```python
from build123d import *

# Parameters (mm, degrees)
SKETCH1_W           = 13
SKETCH1_H           = 8.9
BOSS_EXTRUDE1_DEPTH = 2
SKETCH2_R           = 1.75
CUT_EXTRUDE4_DEPTH  = 9.127268914
SKETCH3_R           = 2.95
CUT_EXTRUDE9_DEPTH  = 0.5
CHAMFER1_SIZE       = 0.5
FILLET2_R           = 2


with BuildPart() as part:
    # Sketch1 → Boss-Extrude1 (new body)
    with BuildSketch(Plane.XY):
        Rectangle(SKETCH1_W, SKETCH1_H)
    extrude(amount=BOSS_EXTRUDE1_DEPTH)

    # Sketch2 → Cut-Extrude4 (cut, through all)
    with BuildSketch(Plane.XY.offset(2)):
        with Locations((-0.4, 1.45)):
            Circle(SKETCH2_R)
    extrude(amount=-CUT_EXTRUDE4_DEPTH, mode=Mode.SUBTRACT)

    # Sketch3 → Cut-Extrude9 (cut)
    with BuildSketch(Plane.XY.offset(2)):
        with Locations((-0.4, 1.45)):
            Circle(SKETCH3_R)
    extrude(amount=-CUT_EXTRUDE9_DEPTH, mode=Mode.SUBTRACT)

    # Chamfer1
    chamfer1_edges = [part.edges().sort_by_distance(p)[0] for p in [
        (-2.15, 1.45, 0),
        (0, -4.45, 0),
        (-6.5, 0, 0),
        (0, 4.45, 0),
        (6.5, 0, 0),
    ]]
    chamfer(chamfer1_edges, length=CHAMFER1_SIZE)

    # Fillet2
    # the kernel refuses this fillet: 2 mm, written as the material it takes off along each edge
    with BuildSketch(Plane(origin=(-6.5, 4.45, -4.5), x_dir=(0, -1, 0), z_dir=(0, 0, 1)), Plane(origin=(-6.5, -4.45, -4.5), x_dir=(1, 0, 0), z_dir=(0, 0, 1))) as fillet2_piece_1:
        with BuildLine():
            CenterArc((FILLET2_R, FILLET2_R), FILLET2_R, 180, 90)
            Line((0, FILLET2_R), (0, 0))
            Line((0, 0), (FILLET2_R, 0))
        make_face()
    extrude(amount=11.5, mode=Mode.SUBTRACT)
    with BuildSketch(Plane(origin=(6.5, 4.45, -4.5), x_dir=(0, -1, 0), z_dir=(0, 0, 1)), Plane(origin=(6.5, -4.45, -4.5), x_dir=(-1, 0, 0), z_dir=(0, 0, 1))) as fillet2_piece_2:
        with BuildLine():
            CenterArc((FILLET2_R, -FILLET2_R), FILLET2_R, 90, 90)
            Line((0, -FILLET2_R), (0, 0))
            Line((0, 0), (FILLET2_R, 0))
        make_face()
    extrude(amount=11.5, mode=Mode.SUBTRACT)


solid = part.part
```
Design review of the part built by this model. Coordinates are the model's own, in mm. Give positions to 0.01 mm unless a question says otherwise; leave off trailing zeros. Loops run counter-clockwise (first coordinate to the right, second up) from the corner with the lowest first, then second, coordinate; pieces in that order, holes last. Notation, with made-up numbers: M 34,77.5 L 92,77.5 A14 ccw 92,85.5 Z; hole C 89.5,-13 d7. An arc over 180 degrees is marked long. Return JSON: item names as keys, results as strings. Group by question number.
Item 1: We need section C-C (x = -0.4). Give the boundary of the cut face in (y, z).
Item 2: We need section A-A (y = 1.45). Give the boundary of the cut face in (x, z).
Item 3: Mouldability with a two-part tool opening along X and no side actions: class faces 1 (the cylindrical face through (5.93, 3.85, 1.21)), 2 (the flat face through (1, 0, 1.5)), 3 (the flat face through (0, -4.45, 1)), 4 (the cylindrical face through (-1.04, -1.43, 1.75)) as released by +X, released by -X, zero draft, split by the parting line, or undercut.
Item 4: We need section B-B (z = 1). Give the boundary of the cut face in (x, y), and give its area (3 significant figures).
Item 5: Insertion check: pin 1 Ø4 at (x, y) = (-0.4, 1.45) entering from -Z; pin 2 Ø4.5 at (x, y) = (0, 1) entering from +Z. Each pin has a flat end and moves straight along its axis. Give the tip position at first contact, or say it passes through.
Item 6: For probe 1 along Y at (x, z) = (-0.4, 1.15); probe 2 along Z at (x, y) = (-3, 0.5); probe 3 along Y at (x, z) = (1.25, 0.3), list the stretches that pass through material, from the lowest coordinate up.
Item 7: We need section D-D (z = 1.7). Give the boundary of the cut face in (x, y), and give its area (3 significant figures).
Output:
{
 "1": {"outline": "M -4.45,0.5 L -3.95,0 L -0.8,0 L -0.3,0.5 L -0.3,1.5 L -1.5,1.5 L -1.5,2 L -4.45,2 Z; M 3.2,0.5 L 3.7,0 L 3.95,0 L 4.45,0.5 L 4.45,2 L 4.4,2 L 4.4,1.5 L 3.2,1.5 Z"},
 "2": {"outline": "M -6.5,0.5 L -6,0 L -2.65,0 L -2.15,0.5 L -2.15,1.5 L -3.35,1.5 L -3.35,2 L -6.5,2 Z; M 1.35,0.5 L 1.85,0 L 6,0 L 6.5,0.5 L 6.5,2 L 2.55,2 L 2.55,1.5 L 1.35,1.5 Z"},
 "3": {"face 1": "released by +X", "face 2": "undercut", "face 3": "zero draft", "face 4": "undercut"},
 "4": {"outline": "M -6.5,-2.45 A2 ccw -4.5,-4.45 L 4.5,-4.45 A2 ccw 6.5,-2.45 L 6.5,2.45 A2 ccw 4.5,4.45 L -4.5,4.45 A2 ccw -6.5,2.45 Z; hole C -0.4,1.45 d3.5", "area": "103 mm^2"},
 "5": {"pin 1": "stops at z = 0.25", "pin 2": "stops at z = 1.5"},
 "6": {"probe 1": "y = -4.45 to -0.3, 3.2 to 4.45", "probe 2": "z = 0 to 1.5", "probe 3": "y = -4.25 to 0.41, 2.49 to 4.25"},
 "7": {"outline": "M -6.5,-2.45 A2 ccw -4.5,-4.45 L 4.5,-4.45 A2 ccw 6.5,-2.45 L 6.5,2.45 A2 ccw 4.5,4.45 L -4.5,4.45 A2 ccw -6.5,2.45 Z; hole C -0.4,1.45 d5.9", "area": "84.9 mm^2"}
}
